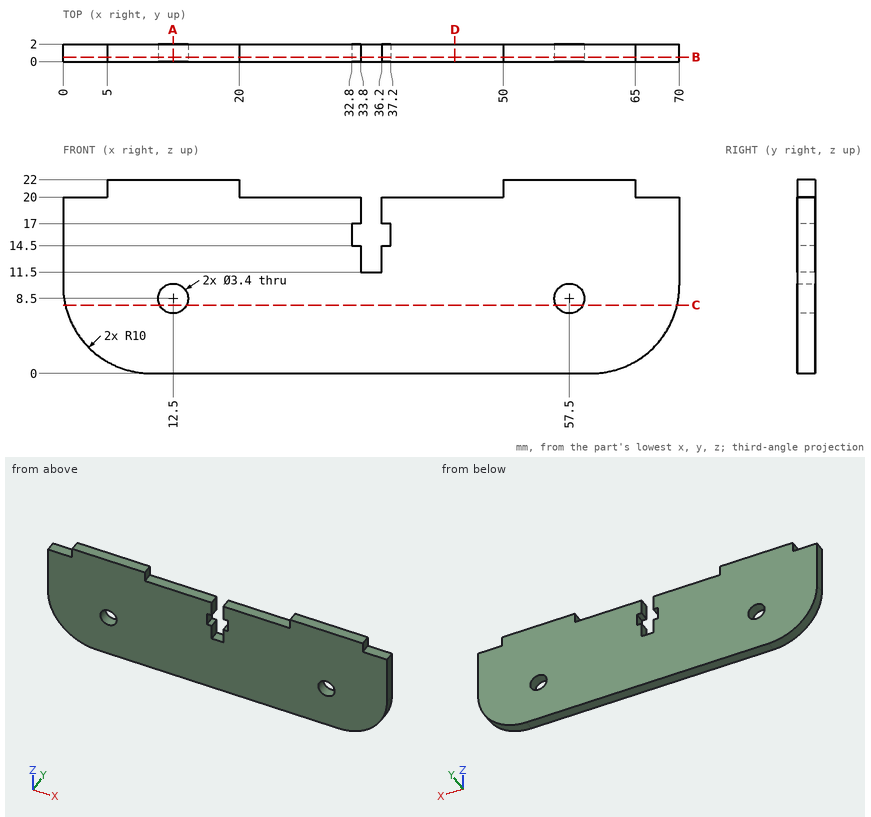
Job drawing, mm, ordinate dimensions from the low corner. One solid piece. Give positions to 0.01 mm unless a question says otherwise; leave off trailing zeros. Write each loop counter-clockwise with the first axis right and the second up, starting at its lowest first coordinate (ties: lowest second). Pieces come first, ordered by that corner, then holes. Notation, with made-up numbers: (57.25, -11) - (83.25, -11) arc R27 ccw to (83.25, 17) - close; hole circle Ø2 at (77, 83). An arc over 180 degrees is marked (long way). Answer as CSV lines item,"result".
1. Drill centre lines: L1, parallel to X at y = 0.7, z = 20.5; L2, parallel to X at y = 1.6, z = 7.75; L3, parallel to X at y = 1.3, z = 8.5. Where is each one in solid material? Low to high. Write a range as [from, to].
Responses:
L1,"x = [5, 20], [50, 65]"
L2,"x = [0.26, 10.97], [14.03, 55.97], [59.03, 69.74]"
L3,"x = [0.11, 10.8], [14.2, 55.8], [59.2, 69.89]"
2. Band-saw the part on D-D (x = 44.5). Write the cut outline in (y, z).
Responses:
outline,"(0, 0) - (2, 0) - (2, 20) - (0, 20) - close"
3. Band-saw the part on B-B (y = 0.5). Write the cut outline in (x, z).
Responses:
outline,"(0, 10) arc R10 ccw to (10, 0) - (60, 0) arc R10 ccw to (70, 10) - (70, 20) - (65, 20) - (65, 22) - (50, 22) - (50, 20) - (36.2, 20) - (36.2, 17) - (37.2, 17) - (37.2, 14.5) - (36.2, 14.5) - (36.2, 11.5) - (33.8, 11.5) - (33.8, 14.5) - (32.8, 14.5) - (32.8, 17) - (33.8, 17) - (33.8, 20) - (20, 20) - (20, 22) - (5, 22) - (5, 20) - (0, 20) - close; hole circle Ø3.4 at (12.5, 8.5); hole circle Ø3.4 at (57.5, 8.5)"
4. Pin check, flat tips, straight feed: pin 1 (1 mm diameter, centred on y = 1, z = 21, fed in from -X); pin 2 (0.6 mm diameter, centred on x = 2.5, y = 1, fed in from +Z). Stop position of each tip, or through.
Responses:
pin 1,"stops at x = 5"
pin 2,"stops at z = 20"
5. Band-saw the part on C-C (z = 7.75). Write the cut outline in (x, y).
Responses:
outline,"(0.26, 0) - (10.97, 0) - (10.97, 2) - (0.26, 2) - close; (14.03, 0) - (55.97, 0) - (55.97, 2) - (14.03, 2) - close; (59.03, 0) - (69.74, 0) - (69.74, 2) - (59.03, 2) - close"
6. Band-saw the part on A-A (x = 12.5). Write the cut outline in (y, z).
Responses:
outline,"(0, 0) - (2, 0) - (2, 6.8) - (0, 6.8) - close; (0, 10.2) - (2, 10.2) - (2, 22) - (0, 22) - close"
